```python
from build123d import *

# Parameters (mm, degrees)
BOSS_EXTRUDE1_DEPTH = 19.05
FILLET1_R           = 3
FILLET2_R           = 4.5875


with BuildPart() as part:
    # Sketch1 → Boss-Extrude1 (new body)
    with BuildSketch(Plane.XY):
        Polygon((-100, 0), (0, 0), (0, 110), (-150, 110), (-150, 95), (-148.4125, 95), (-148.4125, 108.4125), (-1.5875, 108.4125), (-1.5875, 1.5875), (-100, 1.5875), align=None)
    extrude(amount=BOSS_EXTRUDE1_DEPTH)

    # Fillet1
    fillet1_edges = [part.edges().sort_by_distance(p)[0] for p in [
        (-1.5875, 1.5875, 9.525),
        (-1.5875, 108.4125, 9.525),
        (-148.4125, 108.4125, 9.525),
    ]]
    fillet(fillet1_edges, radius=FILLET1_R)

    # Fillet2
    fillet2_edges = [part.edges().sort_by_distance(p)[0] for p in [
        (-150, 110, 9.525),
        (0, 110, 9.525),
        (0, 0, 9.525),
    ]]
    fillet(fillet2_edges, radius=FILLET2_R)


solid = part.part
```
The listing builds one solid part. Answer for the finished solid, in the listing's coordinates (mm). A direction names the side the tool comes from. Round coordinates to 2 decimals unless told otherwise and drop trailing zeros. Order: outer loops, then holes, each group sorted by start corner. A loop starts at its lowest first (then second) coordinate and runs counter-clockwise, first axis right, second up. Notation, with made-up numbers: (41.25, 39.5) - (82.25, 39.5) arc R10 cw to (82.25, 49.5) - close; hole circle Ø3 at (54.25, 38.25). An arc over 180 degrees is marked (long way). Put each result on its own line as item: value. Start each with the question number.
(1) Find section B-B (y = 103.5). Give the vertices of the cut face in (x, z).
(2) Find section A-A (x = -70.5). Give the vertices of the cut face in (y, z), plus the area to 3 significant figures.
(3) Find section C-C (z = 4.5). Give the vertices of the cut face in (x, y) (1 decimal), plus the area to 3 significant figures.
(4) For faces 4 (the flat face through (-53, 0, 9)), 5 (the cylindrical face through (-1.38, 108.69, 9.66)), 6 (the cylindrical face through (-147.56, 107.51, 9.66)), 7 (the cylindrical face through (-2.49, 107.56, 9.66)), 8 (the flat face through (-52, 1.588, 9)), determine the directions among +Z, -Z, +X, -X, +Y, -Y from which every point of the face is accessible in a straight line to the end or side of a thin tool.
(5) Determine the mould class of faces 1 (the flat face through (0, 54, 9)), 2 (the cylindrical face through (-1.31, 1.38, 9.66)), 3 (the flat face through (-76, 108.412, 9)) for opening direction Y: released by +Y, released by -Y, zero draft, split by the parting line, or undercut.
(6) Given P1, Ø0.8, axis at x = -149, z = 8, coming from the -Y side; P2, Ø0.5, axis at y = 1, z = 14, coming from the -X side, each flat-ended and moving along its own axis, determine where each tip first touches the part or whether it passes through.
(7) Find section D-D (y = 83). Give the vertices of the cut face in (x, z).
(8) Straight lines are drawn through the part: probe 1 along Y at (x, z) = (-15, 2); probe 2 along X at (y, z) = (105.5, 9); probe 3 along X at (y, z) = (48, 16). For each, find the intervals that lie inside material, in ascending order. Write a range as from..to.
Reply:
1. outline: (-150, 0) - (-148.41, 0) - (-148.41, 19.05) - (-150, 19.05) - close; (-1.59, 0) - (0, 0) - (0, 19.05) - (-1.59, 19.05) - close
2. outline: (0, 0) - (1.59, 0) - (1.59, 19.05) - (0, 19.05) - close; (108.41, 0) - (110, 0) - (110, 19.05) - (108.41, 19.05) - close
2. area: 60.5 mm^2
3. outline: (-150, 95) - (-148.4, 95) - (-148.4, 105.4) arc R3 cw to (-145.4, 108.4) - (-4.6, 108.4) arc R3 cw to (-1.6, 105.4) - (-1.6, 4.6) arc R3 cw to (-4.6, 1.6) - (-100, 1.6) - (-100, 0) - (-4.6, 0) arc R4.6 ccw to (0, 4.6) - (0, 105.4) arc R4.6 ccw to (-4.6, 110) - (-145.4, 110) arc R4.6 ccw to (-150, 105.4) - close
3. area: 580 mm^2
4. face 4: +Z, -Z, +X, -X, -Y
4. face 5: +Z, -Z, +X, +Y
4. face 6: +Z, -Z, -Y
4. face 7: +Z, -Z
4. face 8: +Z, -Z, -X
5. face 1: zero draft
5. face 2: released by -Y
5. face 3: undercut
6. P1: y = 95
6. P2: x = -100
7. outline: (-1.59, 0) - (0, 0) - (0, 19.05) - (-1.59, 19.05) - close
8. probe 1: 0..1.59, 108.41..110
8. probe 2: -150..-148.41, -1.59..0
8. probe 3: -1.59..0
